The model under review builds one solid part; all positions refer to its coordinate system, in mm. Face numbers are marked on the shaded views. A direction names the side the tool comes from. Round coordinates to 2 decimals unless told otherwise and drop trailing zeros. Return JSON: item names as keys, results as strings. Group by question number.
Q1. To check wall thickness, follow line 1 along Z through (x, y) = (4.5, -2.5); line 2 along Z through (x, y) = (3.5, -5.5); line 3 along X through (y, z) = (-3.5, 5). State the ranges of each line that lie inside material, in increasing order.
Q2. Clearance check with flat-ended pins moving along their axes: pin 1 Ø2 at (x, z) = (1.5, 16) entering from -Y; pin 2 Ø1 at (x, y) = (2.5, -3) entering from +Z; pin 3 Ø5 at (x, y) = (-3.5, 1) entering from +Z. State where each tip first meets the part, or that it passes through.
Q3. For the marked faces 3 and 4, list the 3-axis set-ups (+Z, -Z, +X, -X, +Y, -Y) from which the entire face can be reached by the end or side of a thin tool; tool diameter is ignored.
Q4. Draft analysis for pull direction Y (two halves, no side actions). For the marked faces 1 and 2, state which applies: pulls with the +Y half, pulls with the -Y half, needs draft (parallel to the pull), parting line crosses it, or undercut.
from build123d import *

# Parameters (mm, degrees)
SKETCH2_R           = 22.5
BOSS_EXTRUDE1_DEPTH = 5
FILLET1_R           = 5
SKETCH3_R           = 12
SKETCH3_R_2         = 6
CUT_EXTRUDE1_DEPTH  = 2
SKETCH4_R           = 2.25
CUT_EXTRUDE2_DEPTH  = 34.354160228


with BuildPart() as part:
    # Sketch2 → Boss-Extrude1 (new, symmetric)
    with BuildSketch(Plane(origin=(0, 0, 0), x_dir=(0, 0, -1), z_dir=(1, 0, 0))):
        Circle(SKETCH2_R)
    extrude(amount=BOSS_EXTRUDE1_DEPTH, both=True)

    # Fillet1
    fillet1_edges = [part.edges().sort_by_distance(p)[0] for p in [
        (-5, 0, 22.5),
        (5, 0, 22.5),
    ]]
    fillet(fillet1_edges, radius=FILLET1_R - 0.0001)  # a hair under: the kernel refuses the full size

    # Sketch3 → Cut-Extrude1 (cut)
    with BuildSketch(Plane(origin=(5, 0, 0), x_dir=(0, 0, -1), z_dir=(1, 0, 0))):
        Circle(SKETCH3_R)
        Circle(SKETCH3_R_2, mode=Mode.SUBTRACT)
    cut_extrude1 = extrude(amount=-CUT_EXTRUDE1_DEPTH, mode=Mode.SUBTRACT)

    # Mirror1: Cut-Extrude1 across plane
    add(cut_extrude1.mirror(Plane(origin=(0, 0, 0), x_dir=(0, 0, 1), z_dir=(1, 0, 0))), mode=Mode.SUBTRACT)

    # Sketch4 → Cut-Extrude2 (cut, through all)
    with BuildSketch(Plane(origin=(5, 0, 0), x_dir=(0, 0, -1), z_dir=(1, 0, 0))):
        Circle(SKETCH4_R)
    extrude(amount=-CUT_EXTRUDE2_DEPTH, mode=Mode.SUBTRACT)


solid = part.part
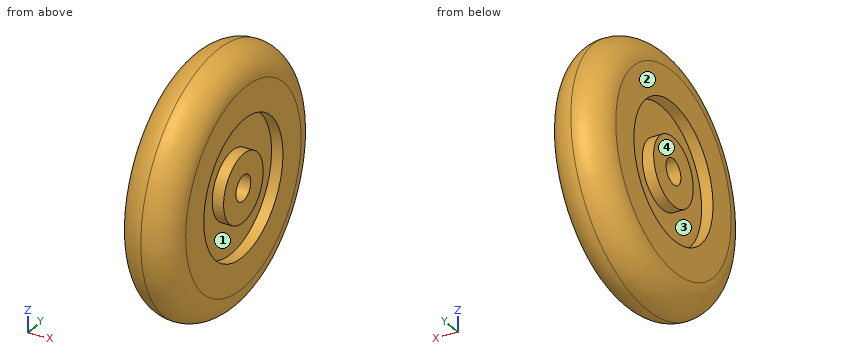
Values:
{
 "1": {"line 1": "z = -19.52 to -11.74, -5.45 to 5.45, 11.74 to 19.52", "line 2": "z = -20.34 to -10.67, -2.4 to 2.4, 10.67 to 20.34", "line 3": "x = -3 to 3"},
 "2": {"pin 1": "stops at y = -16.53", "pin 2": "stops at z = 21.89", "pin 3": "stops at z = 22.38"},
 "3": {"face 3": "-X", "face 4": "+Z, -Z, -X, +Y, -Y"},
 "4": {"face 1": "undercut", "face 2": "needs draft"}
}
